Check sheet for the modelled part. Datum: model origin and axes. Units: mm. Face numbers are marked on the shaded views. Round coordinates to 2 decimals unless told otherwise and drop trailing zeros. Order: outer loops, then holes, each group sorted by start corner. A loop starts at its lowest first (then second) coordinate and runs counter-clockwise, first axis right, second up. Notation, with made-up numbers: (57.5, -31) -> (96.5, -31) arc R26 ccw to (96.5, 0) -> close; hole circle Ø6 at (61.25, 2). An arc over 180 degrees is marked (long way). Answer in a Markdown table with one row per item. Add a question column.
1. Draft check along Y on the marked faces 1 and 2. Enter one of: +Y half, -Y half, draft (parallel to the pull), parting line (faces both ways), or undercut.
2. Sectioned sample at B-B, the plane y = 9.5. Record the boundary of the cut face in (x, z).
3. Material ranges on L1, parallel to Z at x = 10, y = 80; L2, parallel to X at y = 4.5, z = -0.5; L3, parallel to Z at x = 2, y = 23.5, recorded low to high. Write a range as from..to.
4. Depth check by flat-ended pin: P1, Ø8, axis at x = 2, z = 11.5, coming from the +Y side; P2, Ø3, axis at x = 3, y = 31, coming from the -Z side; P3, Ø3, axis at y = 37.5, z = 0.5, coming from the +X side. Enter the tip coordinate at first touch or a pass-through.
5. Sectioned sample at A-A, the plane y = 44.5. Record the boundary of the cut face in (x, z).
```python
from build123d import *


with BuildPart() as part:
    # Sketch1 → Revolve1 (revolve)
    with BuildSketch(Plane.XY, mode=Mode.PRIVATE) as revolve1_sk:
        with BuildLine():
            Line((-15, 0), (0, 0))
            Line((0, 0), (0, 83))
            Line((0, 83), (-2, 83))
            ThreePointArc((-2, 83), (-7.394335397, 82.257693837), (-12.5, 80.365060283))
            Line((-12.5, 80.365060283), (-12.5, 79.365060283))
            Line((-12.5, 79.365060283), (-7.5, 64.365060283))
            Line((-7.5, 64.365060283), (-7.5, 63.365060283))
            ThreePointArc((-7.5, 63.365060283), (-8, 61.085924924), (-6, 59.884068865))
            ThreePointArc((-6, 59.884068865), (-4.460944967, 38.549386799), (-8, 17.454068865))
            ThreePointArc((-8, 17.454068865), (-9.414213562, 16.868282427), (-10, 15.454068865))
            Line((-10, 15.454068865), (-10, 14.454068865))
            ThreePointArc((-10, 14.454068865), (-14, 10.520343653), (-13, 5))
            Line((-13, 5), (-15, 3))
            Line((-15, 3), (-15, 0))
        make_face()
        with BuildLine():
            Line((-2, 83), (0, 83))
            Line((0, 83), (0, 85))
            ThreePointArc((0, 85), (-1.414213562, 84.414213562), (-2, 83))
        make_face()
    revolve(revolve1_sk.sketch.rotate(Axis((0, 0, 0), (0, 1, 0)), 270), axis=Axis((0, 0, 0), (0, 1, 0)))


solid = part.part
```
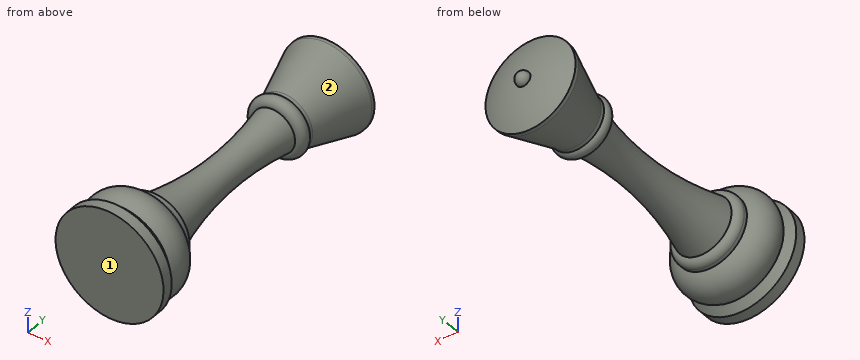
Answer key:
| question | item | result |
|---|---|---|
| 1 | face 1 | -Y half |
| 1 | face 2 | undercut |
| 2 | outline | circle Ø28.46 at (0, 0) |
| 3 | L1 | z = -7.5..7.5 |
| 3 | L2 | x = -13.49..13.49 |
| 3 | L3 | z = -6.13..6.13 |
| 4 | P1 | stops at y = 82.19 |
| 4 | P2 | stops at z = -4.96 |
| 4 | P3 | stops at x = 4.61 |
| 5 | outline | circle Ø8.75 at (0, 0) |
